Source: CAD feature listing. Evaluate the final solid. Frame: model axes, mm. Face numbers are marked on the shaded views. Round coordinates to 2 decimals unless told otherwise and drop trailing zeros. Loops run counter-clockwise (first coordinate to the right, second up) from the corner with the lowest first, then second, coordinate; pieces in that order, holes last. Notation, with made-up numbers: M 24,56 L 41,56 A23 cw 41,76 Z; hole C -31.75,3 d4. An arc over 180 degrees is marked long. Answer as a JSON object with one key per item and string values.
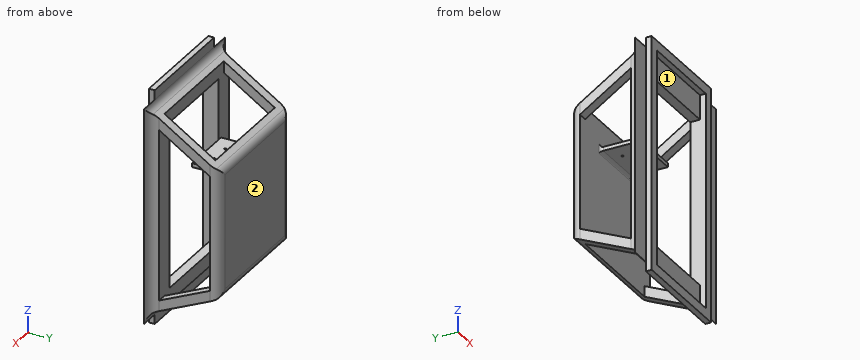
from build123d import *

# Parameters (mm, degrees)
SKETCH1_W           = 200
SKETCH1_H           = 150
BOSS_EXTRUDE1_DEPTH = 280
SKETCH2_W           = 44
SKETCH2_H           = 60
SKETCH2_W_2         = 34
SKETCH2_H_2         = 72.5
CUT_EXTRUDE1_DEPTH  = 280
CUT_EXTRUDE5_DEPTH  = 200
CUT_EXTRUDE8_DEPTH  = 44
CUT_EXTRUDE9_DEPTH  = 44
SKETCH6_W           = 112
SKETCH6_H           = 52.5
CUT_EXTRUDE7_DEPTH  = 280
FILLET1_START       = -100
FILLET1_DEPTH       = 200
FILLET1_START_2     = -76
FILLET1_2_DEPTH     = 10
FILLET1_START_3     = 66
FILLET1_3_DEPTH     = 10
FILLET1_START_4     = -66
FILLET1_4_DEPTH     = 132
FILLET1_START_5     = -281
FILLET1_5_DEPTH     = 282
SKETCH8_W           = 211.062900289
SKETCH8_H           = 77.5
CUT_EXTRUDE10_DEPTH = 280
SKETCH10_W          = 112
SKETCH10_H          = 9.821718876
SKETCH10_H_2        = 221.856562249
SKETCH10_H_3        = 9.821718875
BOSS_EXTRUDE2_DEPTH = 6
SKETCH10_4_W        = 92
SKETCH10_4_H        = 171.032653569
CUT_EXTRUDE11_DEPTH = 10
BOSS_EXTRUDE3_START = -110
SKETCH11_W          = 54.725299756
SKETCH11_H          = 39.681004686
SKETCH11_R          = 1.1
BOSS_EXTRUDE3_DEPTH = 4
FILLET2_R           = 3


with BuildPart() as part:
    # Sketch1 → Boss-Extrude1 (new body)
    with BuildSketch(Plane.XY):
        Rectangle(SKETCH1_W, SKETCH1_H)
    extrude(amount=-BOSS_EXTRUDE1_DEPTH)

    # Sketch2 → Cut-Extrude1 (cut)
    with BuildSketch(Plane.XY):
        with Locations((78, -45)):
            Rectangle(SKETCH2_W, SKETCH2_H)
        with Locations((-78, -45)):
            Rectangle(SKETCH2_W, SKETCH2_H)
        with Locations((83, 38.75)):
            Rectangle(SKETCH2_W_2, SKETCH2_H_2)
        with Locations((-83, 38.75)):
            Rectangle(SKETCH2_W_2, SKETCH2_H_2)
    extrude(amount=-CUT_EXTRUDE1_DEPTH, mode=Mode.SUBTRACT)

    # Sketch3 → Cut-Extrude5 (cut)
    with BuildSketch(Plane.ZY.offset(100)):
        Polygon((-280, 2.5), (-274.399041425, 2.5), (-252, 2.5), (-218.971094498, 75), (-280, 75), align=None)
        Polygon((-236.455453487, 12.5), (-168.766953205, 12.5), (-60.438488841, 12.5), (-94.602997447, 65), (-144.84946991, 65), (-212.537970192, 65), align=None)
        Polygon((-89.179559504, 75), (-42, 2.5), (-5.600958575, 2.5), (0, 2.5), (0, 75), align=None)
    extrude(amount=-CUT_EXTRUDE5_DEPTH, mode=Mode.SUBTRACT)

    # Sketch5 → Cut-Extrude8 (cut)
    with BuildSketch(Plane.ZY.offset(100)):
        Polygon((-264.773291637, -7.125749789), (-270.374250211, -15), (-140, -15), (-140, -7.125749789), align=None)
        Polygon((-15.226708363, -7.125749789), (-140, -7.125749789), (-140, -15), (-9.625749789, -15), align=None)
    extrude(amount=-CUT_EXTRUDE8_DEPTH, mode=Mode.SUBTRACT)

    # Sketch7 → Cut-Extrude9 (cut)
    with BuildSketch(Plane(origin=(100, 0, 0), x_dir=(0, 0, -1), z_dir=(1, 0, 0))):
        Polygon((9.625749789, -15), (15.226708363, -7.125749789), (264.773291637, -7.125749789), (270.374250211, -15), align=None)
    extrude(amount=-CUT_EXTRUDE9_DEPTH, mode=Mode.SUBTRACT)

    # Sketch6 → Cut-Extrude7 (cut)
    with BuildSketch(Plane.XY):
        with Locations((0, 38.75)):
            Rectangle(SKETCH6_W, SKETCH6_H)
    extrude(amount=-CUT_EXTRUDE7_DEPTH, mode=Mode.SUBTRACT)

    # Fillet1: read off the stored shape, not the designer's step
    # Fillet1 outline → Fillet1 (cut)
    with BuildSketch(Plane.YZ.offset(FILLET1_START)):
        with BuildLine():
            Line((-75, 0), (-75, -10))
            ThreePointArc((-75, -10), (-72.071067812, -2.928932188), (-65, 0))
            Line((-65, 0), (-75, 0))
        make_face()
        with BuildLine():
            ThreePointArc((-65, -280), (-72.071067812, -277.071067812), (-75, -270))
            Line((-75, -270), (-75, -280))
            Line((-75, -280), (-65, -280))
        make_face()
        with BuildLine():
            Line((2.5, 0), (-7.5, 0))
            ThreePointArc((-7.5, 0), (-0.428932188, -2.928932188), (2.5, -10))
            Line((2.5, -10), (2.5, 0))
        make_face()
        with BuildLine():
            ThreePointArc((2.5, -270), (-0.428932188, -277.071067812), (-7.5, -280))
            Line((-7.5, -280), (2.5, -280))
            Line((2.5, -280), (2.5, -270))
        make_face()
        with BuildLine():
            Line((75, -89.179559504), (70.454316835, -86.221444616))
            ThreePointArc((70.454316835, -86.221444616), (73.790425711, -89.835564613), (75, -94.602997447))
            Line((75, -94.602997447), (75, -89.179559504))
        make_face()
        with BuildLine():
            ThreePointArc((75, -212.537970192), (73.410042611, -217.948255145), (69.145763344, -221.638115591))
            Line((69.145763344, -221.638115591), (75, -218.971094498))
            Line((75, -218.971094498), (75, -212.537970192))
        make_face()
    extrude(amount=FILLET1_DEPTH, mode=Mode.SUBTRACT)

    # Fillet1 2 outline → Fillet1 2 (add)
    with BuildSketch(Plane.YZ.offset(FILLET1_START_2)):
        with BuildLine():
            ThreePointArc((7.045683165, -44.958114888), (3.709574289, -41.343994891), (2.5, -36.576562057))
            Line((2.5, -36.576562057), (2.5, -258.433124306))
            ThreePointArc((2.5, -258.433124306), (4.089957389, -253.022839352), (8.354236656, -249.332978906))
            Line((8.354236656, -249.332978906), (69.145763344, -221.638115591))
            ThreePointArc((69.145763344, -221.638115591), (73.410042611, -217.948255145), (75, -212.537970192))
            Line((75, -212.537970192), (75, -94.602997447))
            ThreePointArc((75, -94.602997447), (73.790425711, -89.835564613), (70.454316835, -86.221444616))
            Line((70.454316835, -86.221444616), (7.045683165, -44.958114888))
        make_face()
    extrude(amount=FILLET1_2_DEPTH)

    # Fillet1 3 outline → Fillet1 3 (add)
    with BuildSketch(Plane.YZ.offset(FILLET1_START_3)):
        with BuildLine():
            ThreePointArc((7.045683165, -44.958114888), (3.709574289, -41.343994891), (2.5, -36.576562057))
            Line((2.5, -36.576562057), (2.5, -258.433124306))
            ThreePointArc((2.5, -258.433124306), (4.089957389, -253.022839352), (8.354236656, -249.332978906))
            Line((8.354236656, -249.332978906), (69.145763344, -221.638115591))
            ThreePointArc((69.145763344, -221.638115591), (73.410042611, -217.948255145), (75, -212.537970192))
            Line((75, -212.537970192), (75, -94.602997447))
            ThreePointArc((75, -94.602997447), (73.790425711, -89.835564613), (70.454316835, -86.221444616))
            Line((70.454316835, -86.221444616), (7.045683165, -44.958114888))
        make_face()
    extrude(amount=FILLET1_3_DEPTH)

    # Fillet1 4 outline → Fillet1 4 (add)
    with BuildSketch(Plane.YZ.offset(FILLET1_START_4)):
        with BuildLine():
            ThreePointArc((7.045683165, -44.958114888), (3.709574289, -41.343994891), (2.5, -36.576562057))
            Line((2.5, -36.576562057), (2.5, -42))
            Line((2.5, -42), (7.045683165, -44.958114888))
        make_face()
        with BuildLine():
            Line((2.5, -252), (2.5, -258.433124306))
            ThreePointArc((2.5, -258.433124306), (4.089957389, -253.022839352), (8.354236656, -249.332978906))
            Line((8.354236656, -249.332978906), (2.5, -252))
        make_face()
    extrude(amount=FILLET1_4_DEPTH)

    # Fillet1 5 outline → Fillet1 5 (cut)
    with BuildSketch(Plane.XY.offset(FILLET1_START_5)):
        with BuildLine():
            ThreePointArc((56, 75), (63.071067812, 72.071067812), (66, 65))
            Line((66, 65), (66, 12.5))
            ThreePointArc((66, 12.5), (68.928932188, 5.428932188), (76, 2.5))
            Line((76, 2.5), (76, 75))
            Line((76, 75), (56, 75))
        make_face()
        with BuildLine():
            ThreePointArc((-66, 65), (-63.071067812, 72.071067812), (-56, 75))
            Line((-56, 75), (-76, 75))
            Line((-76, 75), (-76, 2.5))
            ThreePointArc((-76, 2.5), (-68.928932188, 5.428932188), (-66, 12.5))
            Line((-66, 12.5), (-66, 65))
        make_face()
        with BuildLine():
            Line((100, 2.5), (90, 2.5))
            ThreePointArc((90, 2.5), (97.071067812, -0.428932188), (100, -7.5))
            Line((100, -7.5), (100, 2.5))
        make_face()
        with BuildLine():
            Line((-90, 2.5), (-100, 2.5))
            Line((-100, 2.5), (-100, -7.5))
            ThreePointArc((-100, -7.5), (-97.071067812, -0.428932188), (-90, 2.5))
        make_face()
        with BuildLine():
            Line((56, -75), (56, -65))
            ThreePointArc((56, -65), (53.071067812, -72.071067812), (46, -75))
            Line((46, -75), (56, -75))
        make_face()
        with BuildLine():
            ThreePointArc((-46, -75), (-53.071067812, -72.071067812), (-56, -65))
            Line((-56, -65), (-56, -75))
            Line((-56, -75), (-46, -75))
        make_face()
    extrude(amount=FILLET1_5_DEPTH, mode=Mode.SUBTRACT)

    # Sketch8 → Cut-Extrude10 (cut)
    with BuildSketch(Plane.XY):
        with Locations((0.683956476, -36.25)):
            Rectangle(SKETCH8_W, SKETCH8_H)
    extrude(amount=-CUT_EXTRUDE10_DEPTH, mode=Mode.SUBTRACT)

    # Sketch10 → Boss-Extrude2 (add)
    # profile 1 of 3: a face of its own
    with BuildSketch(Plane.XZ.offset(-2.5)):
        with Locations((0, -31.665702619)):
            Rectangle(SKETCH10_W, SKETCH10_H)
    # profile 2 of 3: a face of its own
    with BuildSketch(Plane.XZ.offset(-2.5)):
        with Locations((0, -147.504843182)):
            Rectangle(SKETCH10_W, SKETCH10_H_2)
        Polygon((-46, -61.988516397), (-46, -36.754843181), (46, -36.754843181), (46, -61.988516397), (46, -233.021169966), (46, -258.254843181), (-46, -258.254843181), (-46, -233.021169966), align=None, mode=Mode.SUBTRACT)
    # profile 3 of 3: a face of its own
    with BuildSketch(Plane.XZ.offset(-2.5)):
        with Locations((0, -263.343983744)):
            Rectangle(SKETCH10_W, SKETCH10_H_3)
    extrude(amount=BOSS_EXTRUDE2_DEPTH)

    # Sketch10<4> → Cut-Extrude11 (cut)
    with BuildSketch(Plane.XZ.offset(-2.5)):
        with Locations((0, -147.504843182)):
            Rectangle(SKETCH10_4_W, SKETCH10_4_H)
    extrude(amount=-CUT_EXTRUDE11_DEPTH, mode=Mode.SUBTRACT)

    # Sketch11 → Boss-Extrude3 (add)
    with BuildSketch(Plane.XY.offset(BOSS_EXTRUDE3_START)):
        with Locations((0, 45.159497657)):
            Rectangle(SKETCH11_W, SKETCH11_H)
        with Locations((-10.5, 51.409497657)):
            Circle(SKETCH11_R, mode=Mode.SUBTRACT)
        with Locations(Location((10.5, 51.409497657, 0), (0, 0, 180))):
            Circle(SKETCH11_R, mode=Mode.SUBTRACT)
        with Locations((10.5, 38.909497657)):
            Circle(SKETCH11_R, mode=Mode.SUBTRACT)
        with Locations(Location((-10.5, 38.909497657, 0), (0, 0, 180))):
            Circle(SKETCH11_R, mode=Mode.SUBTRACT)
    extrude(amount=-BOSS_EXTRUDE3_DEPTH)

    # Fillet2
    fillet2_edges = [part.edges().sort_by_distance(p)[0] for p in [
        (0, 65, -114),
        (-27.362649878, 65, -112),
        (27.362649878, 65, -112),
        (0, 65, -110),
    ]]
    fillet(fillet2_edges, radius=FILLET2_R)


solid = part.part
Item 1: Section D-D on x = -18. Give the number of separate pieces and of enclosed holes in the cut face, then the cut area to 3 significant figures.
Answer sheet:
{"separate pieces": "3", "enclosed holes": "0", "area": "1,970 mm²"}
Item 2: Section B-B on x = -53. Return the cut outline in (y, z).
Answer sheet:
{"outline": "M -3.5,-268.25 L 2.5,-268.25 L 2.5,-258.43 A10 cw 8.35,-249.33 L 12.5,-247.44 L 12.5,-48.51 L 7.05,-44.96 A10 cw 2.5,-36.58 L 2.5,-26.75 L -3.5,-26.75 Z; M 65,-223.53 L 69.15,-221.64 A10 ccw 75,-212.54 L 75,-94.6 A10 ccw 70.45,-86.22 L 65,-82.67 Z"}
Item 3: Section C-C on y = 19. Return the cut outline in (x, z).
Answer sheet:
{"outline": "M -66,-244.48 L -56,-244.48 L -56,-233.49 L -66,-233.49 Z; M -66,-64.67 L -56,-64.67 L -56,-52.74 L -66,-52.74 Z; M 56,-244.48 L 66,-244.48 L 66,-233.49 L 56,-233.49 Z; M 56,-64.67 L 66,-64.67 L 66,-52.74 L 56,-52.74 Z"}
Item 4: Pull-direction query (Z, two-part tool) for the marked faces 1 and 2; classes: pulls with the +Z half, pulls with the -Z half, needs draft (parallel to the pull), parting line crosses it, or undercut.
Answer sheet:
{"face 1": "undercut", "face 2": "needs draft"}
Item 5: Line query: probe 1 along Y at (x, z) = (-10.5, -112.85); probe 2 along Y at (x, z) = (-48.5, -174.5); probe 3 along Z at (x, y) = (42, 2). Output: solid intervals per line, ascending. Write a range as from..to.
Answer sheet:
{"probe 1": "y = 25.32..37.81, 40.01..50.31, 52.51..75", "probe 2": "y = -3.5..12.5, 65..75", "probe 3": "z = -268.25..-258.25, -36.75..-26.75"}
Item 6: Contact query for flat-ended pins moving along their axis: pin 1 Ø12 at (x, y) = (10, 55.5) entering from -Z; pin 2 Ø4.5 at (y, z) = (39.5, -112.5) entering from -X; pin 3 Ø11 at (x, y) = (5.5, 36) entering from +Z. Output: stop coordinate, or through.
Answer sheet:
{"pin 1": "stops at z = -114", "pin 2": "stops at x = -27.36", "pin 3": "stops at z = -110"}
Item 7: Section A-A on z = -186. Return the cut outline in (x, y).
Answer sheet:
{"outline": "M -76,2.5 L -56,2.5 L -56,-3.5 L -46,-3.5 L -46,12.5 L -66,12.5 A10 cw Z; M -66,65 L 66,65 A10 ccw 56,75 L -56,75 A10 ccw Z; M 46,-3.5 L 56,-3.5 L 56,2.5 L 76,2.5 A10 cw 66,12.5 L 46,12.5 Z"}
